from build123d import *

# Parameters (mm, degrees)
F0_W     = 100
F0_H     = 50
F1_DEPTH = 10
F3_DEPTH = 5
F4_R     = 0.5
F5_DEPTH = 10.001
F6_SIZE  = 2


# Not quite as in the source:
# - a feature names something its author has since deleted; it is built from what else it names


with BuildPart() as f1:
    # F0 (on Top) → F1 (new body)
    with BuildSketch(Plane.XY):
        with Locations((50, 25)):
            Rectangle(F0_W, F0_H)
    extrude(amount=F1_DEPTH)

    # F2 (on face) → F3 (cut)
    with BuildSketch(Plane.XY.offset(10)):
        with BuildLine():
            ThreePointArc((25, 22.3178226352), (26, 21.3178226352), (27, 22.3178226352))
            Line((27, 22.3178226352), (73.0023026059, 22.3178226352))
            ThreePointArc((73.0023026059, 22.3178226352), (73.9660691444, 21.2505758173), (75, 22.25))
            Line((75, 22.25), (75, 27.75))
            ThreePointArc((75, 27.75), (74, 28.75), (73, 27.75))
            Line((73, 27.75), (53, 27.75))
            Line((53, 27.75), (53, 29.75))
            Line((53, 29.75), (47, 29.75))
            Line((47, 29.75), (47, 27.75))
            Line((47, 27.75), (27, 27.75))
            ThreePointArc((27, 27.75), (26, 28.75), (25, 27.75))
            Line((25, 27.75), (25, 22.3178226352))
        make_face()
    extrude(amount=-F3_DEPTH, mode=Mode.SUBTRACT)

    # F4 (on face) → F5 (cut, through all)
    with BuildSketch(Plane.XY.offset(10)):
        with Locations((26.13, 31.7288823426)):
            Circle(F4_R)
        with Locations((28.63, 31.7288823426)):
            Circle(F4_R)
        with Locations((31.13, 31.7288823426)):
            Circle(F4_R)
        with Locations((36.13, 31.7288823426)):
            Circle(F4_R)
        with Locations((41.13, 31.7288823426)):
            Circle(F4_R)
        with Locations((46.13, 31.7288823426)):
            Circle(F4_R)
        with Locations((53.63, 31.7288823426)):
            Circle(F4_R)
        with Locations((61.13, 31.7288823426)):
            Circle(F4_R)
        with Locations((63.63, 31.7288823426)):
            Circle(F4_R)
        with Locations((66.13, 31.7288823426)):
            Circle(F4_R)
        with Locations((68.63, 31.7288823426)):
            Circle(F4_R)
        with Locations((71.13, 31.7288823426)):
            Circle(F4_R)
        with Locations((71.13, 18.3389402926)):
            Circle(F4_R)
        with Locations((61.13, 18.3389402926)):
            Circle(F4_R)
        with Locations((26.13, 18.3389402926)):
            Circle(F4_R)
        with Locations((28.63, 18.3389402926)):
            Circle(F4_R)
        with Locations((31.13, 18.3389402926)):
            Circle(F4_R)
        with Locations((36.13, 18.3389402926)):
            Circle(F4_R)
        with Locations((41.13, 18.3389402926)):
            Circle(F4_R)
        with Locations((46.13, 18.3389402926)):
            Circle(F4_R)
        with Locations((53.63, 18.3389402926)):
            Circle(F4_R)
        with Locations((68.63, 18.3389402926)):
            Circle(F4_R)
        with Locations((26.13, 34.2288823426)):
            Circle(F4_R)
        with Locations((28.63, 34.2288823426)):
            Circle(F4_R)
        with Locations((31.13, 34.2288823426)):
            Circle(F4_R)
        with Locations((36.13, 34.2288823426)):
            Circle(F4_R)
        with Locations((41.13, 34.2288823426)):
            Circle(F4_R)
        with Locations((46.13, 34.2288823426)):
            Circle(F4_R)
        with Locations((53.63, 34.2288823426)):
            Circle(F4_R)
        with Locations((61.13, 34.2288823426)):
            Circle(F4_R)
        with Locations((63.63, 34.2288823426)):
            Circle(F4_R)
        with Locations((66.13, 34.2288823426)):
            Circle(F4_R)
        with Locations((68.63, 34.2288823426)):
            Circle(F4_R)
        with Locations((71.13, 34.2288823426)):
            Circle(F4_R)
        with Locations((41.13, 15.8389402926)):
            Circle(F4_R)
        with Locations((61.13, 15.8389402926)):
            Circle(F4_R)
        with Locations((36.13, 15.8389402926)):
            Circle(F4_R)
        with Locations((53.63, 15.8389402926)):
            Circle(F4_R)
        with Locations((46.13, 15.8389402926)):
            Circle(F4_R)
        with Locations((71.13, 15.8389402926)):
            Circle(F4_R)
        with Locations((31.13, 15.8389402926)):
            Circle(F4_R)
        with Locations((26.13, 15.8389402926)):
            Circle(F4_R)
        with Locations((68.63, 15.8389402926)):
            Circle(F4_R)
        with Locations((28.63, 15.8389402926)):
            Circle(F4_R)
    extrude(amount=-F5_DEPTH, mode=Mode.SUBTRACT)

    # F6
    f6_edges = [f1.edges().sort_by_distance(p)[0] for p in [
        (50, 0, 10),
        (0, 25, 10),
        (50, 50, 10),
        (100, 25, 10),
    ]]
    chamfer(f6_edges, length=F6_SIZE)


solid = f1.part
Could you check a few things on this model? Use its own coordinates, in mm. A direction names the side the tool comes from. Round coordinates to 2 decimals unless told otherwise and drop trailing zeros. Loops run counter-clockwise (first coordinate to the right, second up) from the corner with the lowest first, then second, coordinate; pieces in that order, holes last. Notation, with made-up numbers: (40, -17.75) - (77, -17.75) arc R25 ccw to (77, 7.25) - close; hole circle Ø5 at (55.25, 82). An arc over 180 degrees is marked (long way). Write item = value, one per line.
1) I need wall thicknesses on line 1 along Y through (x, z) = (68.63, 7.75); line 2 along Y through (x, z) = (61.13, 3); line 3 along X through (y, z) = (29, 6.5). Which ranges of each line are inside material? Lowest first, please. Write a range as from..to.
Computed:
line_1 = 0..15.34, 16.34..17.84, 18.84..22.32, 27.75..31.23, 32.23..33.73, 34.73..50
line_2 = 0..15.34, 16.34..17.84, 18.84..31.23, 32.23..33.73, 34.73..50
line_3 = 0..47, 53..100
2) On a 3-axis mill with a long thin cutter (end or side, diameter ignored), from which of +Z, -Z, +X, -X, +Y, -Y can I reach the whole of each face in a straight line? I mean faces 1 (the flat face through (49, 50, 4)), 2 (the cylindrical face through (74.02, 28.75, 7.54)). Say none if no direction works.
Computed:
face_1 = +Z, -Z, +X, -X, +Y
face_2 = +Z
3) If we mould it in two halves opening along Y, with no side actions, what happens to faces 3 (the flat face through (49, 49, 9)), 4 (the flat face through (1, 25, 9)), 5 (the flat face through (50, 22.318, 8))? For each: pulls with the +Y half, pulls with the -Y half, needs draft (parallel to the pull), parting line crosses it, or undercut.
Computed:
face_3 = pulls with the +Y half
face_4 = needs draft
face_5 = undercut
4) Imagine slicing it at A-A (x = 74). Please give me the cut outline in (y, z), and give its area (4 significant figures).
Computed:
outline = (0, 0) - (50, 0) - (50, 8) - (48, 10) - (28.75, 10) - (28.75, 5) - (21.25, 5) - (21.25, 10) - (2, 10) - (0, 8) - close
area = 458.5 mm2
5) Imagine slicing it at B-B (z = 9). Give the number of separate pieces and of enclosed holes in the cut face, and give its area (3 significant figures).
Computed:
separate_pieces = 1
enclosed_holes = 45
area = 4,380 mm2
6) I'm going to push a flat-ended pin straight in: P1, Ø2.5, axis at x = 40, y = 24, coming from the +Z side. Where does the tip first touch, or does it pass through?
Computed:
P1 = 5
